Check sheet for the modelled part. Datum: model origin and axes. Units: mm. A direction names the side the tool comes from. Round coordinates to 2 decimals unless told otherwise and drop trailing zeros. Loops run counter-clockwise (first coordinate to the right, second up) from the corner with the lowest first, then second, coordinate; pieces in that order, holes last. Notation, with made-up numbers: (5, -29) -> (30, -29) arc R21 ccw to (30, 8) -> close; hole circle Ø11 at (-7, -35.75). An arc over 180 degrees is marked (long way). One line per item, written item: value. Start each with the question number.
1. Cross-section at D-D on y = 1. Record the cut outline in (x, z).
2. Material ranges on L1, parallel to Y at x = -6.35, z = 13; L2, parallel to Z at x = -9, y = -25.5; L3, parallel to Y at x = -4, z = 3.5, recorded low to high.
3. Set-up check for faces 4 (the face through (14.35, -15.187, 1.377)), 5 (the face through (4.19, -37.884, 1.377)), 6 (the face through (-27.013, -15.206, 1.377)), 7 (the face through (-25.66, -10.9, 1.38)), 8 (the face through (4, -24, 2.794)): record each of +Z, -Z, +X, -X, +Y, -Y from which the full face is reachable in a straight line by a thin tool's end or side.
4. Cross-section at B-B on z = 9.5. Record the cut outline in (x, y) (3 decimals), then the cut area to 3 significant figures.
5. Cross-section at C-C on z = -2. Record the cut outline in (x, y).
6. Release check for a two-part mould opening along Z. For faces 1 (the face through (-1.168, -19.477, 13.405)), 2 (the face through (-3, -19, 17.794)), 3 (the face through (-16.86, -37.855, 1.377)) record: +Z half, -Z half, draft (parallel to the pull), parting line (faces both ways), or undercut.
7. Cross-section at A-A on x = -6.35. Record the cut outline in (y, z).
8. Go/stop test with flat-tipped pins: pin 1 (2 mm diameter, centred on x = -9, y = -38.5, fed in from +Z); pin 2 (4 mm diameter, centred on y = -19.54, z = 11.91, fed in from +X); pin 3 (12 mm diameter, centred on x = 7, y = -4.5, fed in from -Z). Record where each tip stops, or that it passes through.
from build123d import *

# Parameters (mm, degrees)
BOSS_EXTRUDE1_DEPTH = 2.794
SKETCH3_R           = 7.5
SKETCH3_R_2         = 3.175
BOSS_EXTRUDE2_DEPTH = 15
FILLET1_R           = 3
SKETCH4_R           = 1.5
CUT_EXTRUDE1_DEPTH  = 7.5
SKETCH5_R           = 4
BOSS_EXTRUDE3_DEPTH = 25


with BuildPart() as part:
    # Sketch2 → Boss-Extrude1 (new body)
    with BuildSketch(Plane.XY):
        with BuildLine():
            ThreePointArc((-8.73125, 0), (-8.606730181, 1.469327109), (-8.236722377, 2.896744905))
            ThreePointArc((-8.236722377, 2.896744905), (-6.35, 4.233209924), (-4.463277623, 2.896744905))
            ThreePointArc((-4.463277623, 2.896744905), (-4.093269819, 1.469327109), (-3.96875, 0))
            ThreePointArc((-3.96875, 0), (-3.210786196, -2.33277272), (-1.226411196, -3.774505549))
            ThreePointArc((-1.226411196, -3.774505549), (1.226411196, -3.774505549), (3.210786196, -2.33277272))
            ThreePointArc((3.210786196, -2.33277272), (4.175173652, -1.217253032), (5.313531383, -0.279932907))
            ThreePointArc((5.313531383, -0.279932907), (7.625476277, -0.307697583), (8.366312316, -2.497908084))
            ThreePointArc((8.366312316, -2.497908084), (7.826639788, -3.870198469), (7.063729632, -5.132099984))
            ThreePointArc((7.063729632, -5.132099984), (6.305765829, -7.464872704), (7.063729632, -9.797645424))
            ThreePointArc((7.063729632, -9.797645424), (9.048104632, -11.239378253), (11.500927025, -11.239378253))
            ThreePointArc((11.500927025, -11.239378253), (12.936818887, -10.903756591), (14.408712583, -10.814558567))
            ThreePointArc((14.408712583, -10.814558567), (16.262795625, -12.195947775), (15.574771139, -14.403317789))
            ThreePointArc((15.574771139, -14.403317789), (14.331554842, -15.19631248), (12.972620461, -15.768784912))
            ThreePointArc((12.972620461, -15.768784912), (10.988245461, -17.210517741), (10.230281657, -19.543290461))
            ThreePointArc((10.230281657, -19.543290461), (10.988245461, -21.876063181), (12.972620461, -23.31779601))
            ThreePointArc((12.972620461, -23.31779601), (14.331554842, -23.890268442), (15.574771139, -24.683263133))
            ThreePointArc((15.574771139, -24.683263133), (16.262795625, -26.890633147), (14.408712583, -28.272022355))
            ThreePointArc((14.408712583, -28.272022355), (12.936818887, -28.182824331), (11.500927025, -27.847202669))
            ThreePointArc((11.500927025, -27.847202669), (9.048104632, -27.847202669), (7.063729632, -29.288935498))
            ThreePointArc((7.063729632, -29.288935498), (6.305765829, -31.621708218), (7.063729632, -33.954480938))
            ThreePointArc((7.063729632, -33.954480938), (7.826639788, -35.216382453), (8.366312316, -36.588672839))
            ThreePointArc((8.366312316, -36.588672839), (7.625476277, -38.778883339), (5.313531383, -38.806648015))
            ThreePointArc((5.313531383, -38.806648015), (4.175173652, -37.869327891), (3.210786196, -36.753808202))
            ThreePointArc((3.210786196, -36.753808202), (1.226411196, -35.312075373), (-1.226411196, -35.312075373))
            ThreePointArc((-1.226411196, -35.312075373), (-3.210786196, -36.753808202), (-3.96875, -39.086580922))
            ThreePointArc((-3.96875, -39.086580922), (-4.093269819, -40.555908031), (-4.463277623, -41.983325828))
            ThreePointArc((-4.463277623, -41.983325828), (-6.35, -43.319790846), (-8.236722377, -41.983325828))
            ThreePointArc((-8.236722377, -41.983325828), (-8.606730181, -40.555908031), (-8.73125, -39.086580922))
            ThreePointArc((-8.73125, -39.086580922), (-9.489213804, -36.753808202), (-11.473588804, -35.312075373))
            ThreePointArc((-11.473588804, -35.312075373), (-13.926411196, -35.312075373), (-15.910786196, -36.753808202))
            ThreePointArc((-15.910786196, -36.753808202), (-16.875173652, -37.869327891), (-18.013531383, -38.806648015))
            ThreePointArc((-18.013531383, -38.806648015), (-20.325476277, -38.778883339), (-21.066312316, -36.588672839))
            ThreePointArc((-21.066312316, -36.588672839), (-20.526639788, -35.216382453), (-19.763729632, -33.954480938))
            ThreePointArc((-19.763729632, -33.954480938), (-19.005765829, -31.621708218), (-19.763729632, -29.288935498))
            ThreePointArc((-19.763729632, -29.288935498), (-21.748104632, -27.847202669), (-24.200927025, -27.847202669))
            ThreePointArc((-24.200927025, -27.847202669), (-25.636818887, -28.182824331), (-27.108712583, -28.272022355))
            ThreePointArc((-27.108712583, -28.272022355), (-28.962795625, -26.890633147), (-28.274771139, -24.683263133))
            ThreePointArc((-28.274771139, -24.683263133), (-27.031554842, -23.890268442), (-25.672620461, -23.31779601))
            ThreePointArc((-25.672620461, -23.31779601), (-23.688245461, -21.876063181), (-22.930281657, -19.543290461))
            ThreePointArc((-22.930281657, -19.543290461), (-23.688245461, -17.210517741), (-25.672620461, -15.768784912))
            ThreePointArc((-25.672620461, -15.768784912), (-27.031554842, -15.19631248), (-28.274771139, -14.403317789))
            ThreePointArc((-28.274771139, -14.403317789), (-28.962795625, -12.195947775), (-27.108712583, -10.814558567))
            ThreePointArc((-27.108712583, -10.814558567), (-25.636818887, -10.903756591), (-24.200927025, -11.239378253))
            ThreePointArc((-24.200927025, -11.239378253), (-21.748104632, -11.239378253), (-19.763729632, -9.797645424))
            ThreePointArc((-19.763729632, -9.797645424), (-19.005765829, -7.464872704), (-19.763729632, -5.132099984))
            ThreePointArc((-19.763729632, -5.132099984), (-20.526639788, -3.870198469), (-21.066312316, -2.497908084))
            ThreePointArc((-21.066312316, -2.497908084), (-20.325476277, -0.307697583), (-18.013531383, -0.279932907))
            ThreePointArc((-18.013531383, -0.279932907), (-16.875173652, -1.217253032), (-15.910786196, -2.33277272))
            ThreePointArc((-15.910786196, -2.33277272), (-13.926411196, -3.774505549), (-11.473588804, -3.774505549))
            ThreePointArc((-11.473588804, -3.774505549), (-9.489213804, -2.33277272), (-8.73125, 0))
        make_face()
    extrude(amount=BOSS_EXTRUDE1_DEPTH)

    # Sketch3 → Boss-Extrude2 (add)
    with BuildSketch(Plane.XY.offset(2.794)):
        with Locations((-6.35, -19.543290461)):
            Circle(SKETCH3_R)
        with Locations((-6.35, -19.543290461)):
            Circle(SKETCH3_R_2, mode=Mode.SUBTRACT)
    extrude(amount=BOSS_EXTRUDE2_DEPTH)

    # Fillet1
    fillet1_edges = [part.edges().sort_by_distance(p)[0] for p in [
        (-13.85, -19.543290461, 2.794),
    ]]
    fillet(fillet1_edges, radius=FILLET1_R)

    # Sketch4 → Cut-Extrude1 (cut, symmetric)
    with BuildSketch(Plane(origin=(0, 0, 0), x_dir=(0, 0, -1), z_dir=(1, 0, 0))):
        with Locations((-11.906147171, -19.543290461)):
            Circle(SKETCH4_R)
    extrude(amount=CUT_EXTRUDE1_DEPTH, both=True, mode=Mode.SUBTRACT)

    # Sketch5 → Boss-Extrude3 (add)
    with BuildSketch(Plane(origin=(0, 0, 0), x_dir=(-1, 0, 0), z_dir=(0, 0, -1))):
        with Locations((6.35, -19.543290461)):
            Circle(SKETCH5_R)
    extrude(amount=BOSS_EXTRUDE3_DEPTH)


solid = part.part
Taken from the geometry:
1. outline: (-8.67, 0) -> (-4.03, 0) -> (-4.03, 2.79) -> (-8.67, 2.79) -> close
2. L1: y = -27.04 to -22.72, -16.37 to -12.04
2. L2: z = 0 to 17.79
2. L3: y = -27.78 to -21.68, -17.41 to -11.31
3. face 4: +Z, -Z, +X
3. face 5: +Z, -Z, -Y
3. face 6: +Z, -Z, -X
3. face 7: +Z, -Z, +Y
3. face 8: +Z
4. outline: circle Ø15 at (-6.35, -19.543); hole circle Ø6.35 at (-6.35, -19.543)
4. area: 145 mm2
5. outline: circle Ø8 at (-6.35, -19.54)
6. face 1: undercut
6. face 2: +Z half
6. face 3: draft
7. outline: (-43.32, 0) -> (-23.54, 0) -> (-23.54, -25) -> (-15.54, -25) -> (-15.54, 0) -> (4.23, 0) -> (4.23, 2.79) -> (-9.04, 2.79) arc R3 cw to (-12.04, 5.79) -> (-12.04, 17.79) -> (-16.37, 17.79) -> (-16.37, 2.79) -> (-22.72, 2.79) -> (-22.72, 17.79) -> (-27.04, 17.79) -> (-27.04, 5.79) arc R3 cw to (-30.04, 2.79) -> (-43.32, 2.79) -> close
8. pin 1: stops at z = 2.79
8. pin 2: stops at x = 1.15
8. pin 3: stops at z = 0
